```python
from build123d import *

# Parameters (mm, degrees)
SKETCH_1_W                 = 100
SKETCH_1_H                 = 100
EXTRUDE_1_DEPTH            = 10
CUT_EXTRUDE_2_DEPTH        = 142.774468788
PATTERN_LINEAR_1_COUNT     = 4
PATTERN_LINEAR_1_PITCH     = 22
PATTERN_LINEAR_1_COL_COUNT = 5
PATTERN_LINEAR_1_COL_PITCH = 18


with BuildPart() as part:
    # 草圖1 → 伸長1 (new body)
    with BuildSketch(Plane.XY):
        with Locations((50, 50)):
            Rectangle(SKETCH_1_W, SKETCH_1_H)
    extrude(amount=EXTRUDE_1_DEPTH)

    # 草圖2 → 伸長2 (cut, through all)
    with BuildSketch(Plane.XY.offset(10)):
        Polygon((15.34644344, 17.983526064), (8.935402707, 17.983526064), (5.72988234, 12.431401924), (8.935402707, 6.879277785), (15.34644344, 6.879277785), (18.551963806, 12.431401924), align=None)
    cut_extrude_2 = extrude(amount=-CUT_EXTRUDE_2_DEPTH, mode=Mode.SUBTRACT)

    # 直線複製排列1: 伸長2 ×4
    with Locations(*[(0, i * PATTERN_LINEAR_1_PITCH, 0) for i in range(1, PATTERN_LINEAR_1_COUNT)]):
        add(cut_extrude_2, mode=Mode.SUBTRACT)

    # 直線複製排列1 col: 伸長2 ×5
    with Locations(*[(i * PATTERN_LINEAR_1_COL_PITCH, 0, 0) for i in range(1, PATTERN_LINEAR_1_COL_COUNT)]):
        add(cut_extrude_2, mode=Mode.SUBTRACT)


solid = part.part
```
For this review, take the finished solid that the model builds, in its own axes (mm). Give positions to 0.01 mm unless a question says otherwise; leave off trailing zeros. Write each loop counter-clockwise with the first axis right and the second up, starting at its lowest first coordinate (ties: lowest second). Pieces come first, ordered by that corner, then holes.
Item 1: Take a section at B-B (y = 14.5). Give the boundary of the cut face in (x, z).
Item 2: Wall thickness on probe 1 along Y at (x, z) = (68.5, 2.5); probe 2 along X at (y, z) = (8, 3.5); probe 3 along Y at (x, z) = (62.5, 3.25): over which ranges is each line inside the solid? List them lowest first.
Item 3: Take a section at A-A (x = 66.5). Give the boundary of the cut face in (y, z), and give its area (3 significant figures).
Item 4: Take a section at C-C (z = 4.75). Give the number of separate pieces and of enclosed holes in the cut face, and give its area (3 significant figures).
Item 5: The part is to be moulded in two halves that separate along X. For faces 1 (the face through (49, 51, 10)), 2 (the face through (34.93, 9.62, 5.07)), say which applies: +X half, -X half, draft (parallel to the pull), parting line (faces both ways), or undercut.
Established:
1. outline: (0, 0) - (6.92, 0) - (6.92, 10) - (0, 10) - close; (17.36, 0) - (24.92, 0) - (24.92, 10) - (17.36, 10) - close; (35.36, 0) - (42.92, 0) - (42.92, 10) - (35.36, 10) - close; (53.36, 0) - (60.92, 0) - (60.92, 10) - (53.36, 10) - close; (71.36, 0) - (78.92, 0) - (78.92, 10) - (71.36, 10) - close; (89.36, 0) - (100, 0) - (100, 10) - (89.36, 10) - close
2. probe 1: y = 0 to 6.88, 17.98 to 100
2. probe 2: x = 0 to 8.29, 15.99 to 26.29, 33.99 to 44.29, 51.99 to 62.29, 69.99 to 80.29, 87.99 to 100
2. probe 3: y = 0 to 7.63, 17.23 to 100
3. outline: (0, 0) - (6.88, 0) - (6.88, 10) - (0, 10) - close; (17.98, 0) - (100, 0) - (100, 10) - (17.98, 10) - close
3. area: 889 mm2
4. separate pieces: 1
4. enclosed holes: 8
4. area: 9,150 mm2
5. face 1: draft
5. face 2: undercut
